```python
from build123d import *

# Parameters (mm, degrees)
SKETCH_1_W          = 470
SKETCH_1_H          = 530
SKETCH_1_R          = 7
SKETCH_1_R_2        = 6
SKETCH_1_W_2        = 330
SKETCH_1_H_2        = 390
EXTRUDE_1_DEPTH     = 15
SKETCH_2_W          = 390
SKETCH_2_H          = 450
SKETCH_2_W_2        = 370
SKETCH_2_H_2        = 430
EXTRUDE_2_DEPTH     = 75
CUT_EXTRUDE_1_DEPTH = 514.054577993


with BuildPart() as part:
    # 草图1 → 凸台-拉伸1 (new body)
    with BuildSketch(Plane(origin=(0, 0, 0), x_dir=(0, 0, -1), z_dir=(1, 0, 0))):
        Rectangle(SKETCH_1_W, SKETCH_1_H)
        with Locations((-215, 245)):
            Circle(SKETCH_1_R, mode=Mode.SUBTRACT)
        with Locations((-165, 245)):
            Circle(SKETCH_1_R_2, mode=Mode.SUBTRACT)
        with Locations((-215, 195)):
            Circle(SKETCH_1_R_2, mode=Mode.SUBTRACT)
        with Locations(Location((215, 245, 0), (0, 0, 180))):
            Circle(SKETCH_1_R, mode=Mode.SUBTRACT)
        with Locations(Location((165, 245, 0), (0, 0, 180))):
            Circle(SKETCH_1_R_2, mode=Mode.SUBTRACT)
        with Locations(Location((215, 195, 0), (0, 0, 180))):
            Circle(SKETCH_1_R_2, mode=Mode.SUBTRACT)
        with Locations(Location((-215, -195, 0), (0, 0, 180))):
            Circle(SKETCH_1_R_2, mode=Mode.SUBTRACT)
        with Locations(Location((-165, -245, 0), (0, 0, 180))):
            Circle(SKETCH_1_R_2, mode=Mode.SUBTRACT)
        with Locations(Location((-215, -245, 0), (0, 0, 180))):
            Circle(SKETCH_1_R, mode=Mode.SUBTRACT)
        with Locations((165, -245)):
            Circle(SKETCH_1_R_2, mode=Mode.SUBTRACT)
        with Locations((215, -245)):
            Circle(SKETCH_1_R, mode=Mode.SUBTRACT)
        with Locations((215, -195)):
            Circle(SKETCH_1_R_2, mode=Mode.SUBTRACT)
        with Locations((-215, 0)):
            Circle(SKETCH_1_R_2, mode=Mode.SUBTRACT)
        with Locations(Location((215, 0, 0), (0, 0, 180))):
            Circle(SKETCH_1_R_2, mode=Mode.SUBTRACT)
        Rectangle(SKETCH_1_W_2, SKETCH_1_H_2, mode=Mode.SUBTRACT)
    extrude(amount=EXTRUDE_1_DEPTH)

    # 草图2 → 凸台-拉伸2 (add)
    with BuildSketch(Plane(origin=(15, 0, 0), x_dir=(0, 0, -1), z_dir=(1, 0, 0))):
        Rectangle(SKETCH_2_W, SKETCH_2_H)
        Rectangle(SKETCH_2_W_2, SKETCH_2_H_2, mode=Mode.SUBTRACT)
    extrude(amount=EXTRUDE_2_DEPTH)

    # 草图4 → 切除-拉伸1 (cut, through all)
    with BuildSketch(Plane.XY.offset(195)):
        with BuildLine():
            Line((90, 25), (55, 25))
            ThreePointArc((55, 25), (30, 0), (55, -25))
            Line((55, -25), (90, -25))
            Line((90, -25), (90, 25))
        make_face()
        with BuildLine():
            Line((90, 200), (55, 200))
            ThreePointArc((55, 200), (30, 175), (55, 150))
            Line((55, 150), (90, 150))
            Line((90, 150), (90, 200))
        make_face()
        with BuildLine():
            Line((90, -150), (90, -200))
            Line((90, -200), (55, -200))
            ThreePointArc((55, -200), (30, -175), (55, -150))
            Line((55, -150), (90, -150))
        make_face()
    extrude(amount=-CUT_EXTRUDE_1_DEPTH, mode=Mode.SUBTRACT)


solid = part.part
```
The model under review builds one solid part; all positions refer to its coordinate system, in mm. A direction names the side the tool comes from. Round coordinates to 2 decimals unless told otherwise and drop trailing zeros. Write each loop counter-clockwise with the first axis right and the second up, starting at its lowest first coordinate (ties: lowest second). Pieces come first, ordered by that corner, then holes.
(1) We need section D-D on y = 245. Give the boundary of the cut face in (x, z), and give its area (3 significant figures).
(2) Mouldability with a two-part tool opening along Y and no side actions: class faces 5 (the flat face through (90, -221, 3)), 6 (the flat face through (7, 265, 3)), 7 (the cylindrical face through (7.395, -189.143, 213.699)) as +Y half, -Y half, draft (parallel to the pull), parting line (faces both ways), or undercut.
(3) Machinability: for faces 1 (the flat face through (27, -3, -195)), 2 (the flat face through (52, 215, 3)), 3 (the cylindrical face through (30.006, -175.55, 190.07)), 4 (the flat face through (27, -3, 195)), which of the approach directions +Z, -Z, +X, -X, +Y, -Y give a long, thin tool a straight path to every point of the face, cutting with its end or side? Answer none if there is none.
(4) We need section C-C on z = 83.5. Give the boundary of the cut face in (x, y).
(5) We need section B-B on y = 175. Give the boundary of the cut face in (x, z), and give its area (3 significant figures).
(6) Insertion check: pin 1 (10 mm diameter, centred on x = 38, y = 148, fed in from -Z); pin 2 (14 mm diameter, centred on y = -195, z = 215, fed in from +X); pin 3 (8 mm diameter, centred on x = 80.5, z = -192, fed in from +Y). Each pin has a flat end and moves straight along its axis. Give the tip position at first contact, or say it passes through.
(7) Wall thickness on L1, parallel to Y at x = 11, z = -215; L2, parallel to Z at x = 64.5, y = -45; L3, parallel to Y at x = 49, z = 42: over which ranges is each line inside the solid? List them lowest first.
(8) We need section A-A on z = 215. Give the boundary of the cut face in (x, y).
Findings below:
1. outline: (0, -235) - (15, -235) - (15, -222) - (0, -222) - close; (0, -208) - (15, -208) - (15, -171) - (0, -171) - close; (0, -159) - (15, -159) - (15, 159) - (0, 159) - close; (0, 171) - (15, 171) - (15, 208) - (0, 208) - close; (0, 222) - (15, 222) - (15, 235) - (0, 235) - close
1. area: 6,270 mm2
2. face 5: draft
2. face 6: +Y half
2. face 7: undercut
3. face 1: -Z, +X, +Y, -Y
3. face 2: +X
3. face 3: +Z, -Z, +X
3. face 4: +Z, +X, +Y, -Y
4. outline: (0, -265) - (15, -265) - (15, -225) - (90, -225) - (90, -215) - (15, -215) - (15, -195) - (0, -195) - close; (0, 195) - (15, 195) - (15, 215) - (90, 215) - (90, 225) - (15, 225) - (15, 265) - (0, 265) - close
5. outline: (0, -235) - (15, -235) - (15, -195) - (30, -195) - (30, -185) - (15, -185) - (15, -165) - (0, -165) - close; (0, 165) - (15, 165) - (15, 185) - (30, 185) - (30, 195) - (15, 195) - (15, 235) - (0, 235) - close
5. area: 2,400 mm2
6. pin 1: stops at z = -195
6. pin 2: stops at x = 15
6. pin 3: stops at y = 225
7. L1: y = -265 to -252, -238 to -201, -189 to -6, 6 to 189, 201 to 238, 252 to 265
7. L2: z = -195 to -185, 185 to 195
7. L3: y = -225 to -215, 215 to 225
8. outline: (0, -265) - (15, -265) - (15, -252) - (0, -252) - close; (0, -238) - (15, -238) - (15, -201) - (0, -201) - close; (0, -189) - (15, -189) - (15, -6) - (0, -6) - close; (0, 6) - (15, 6) - (15, 189) - (0, 189) - close; (0, 201) - (15, 201) - (15, 238) - (0, 238) - close; (0, 252) - (15, 252) - (15, 265) - (0, 265) - close
